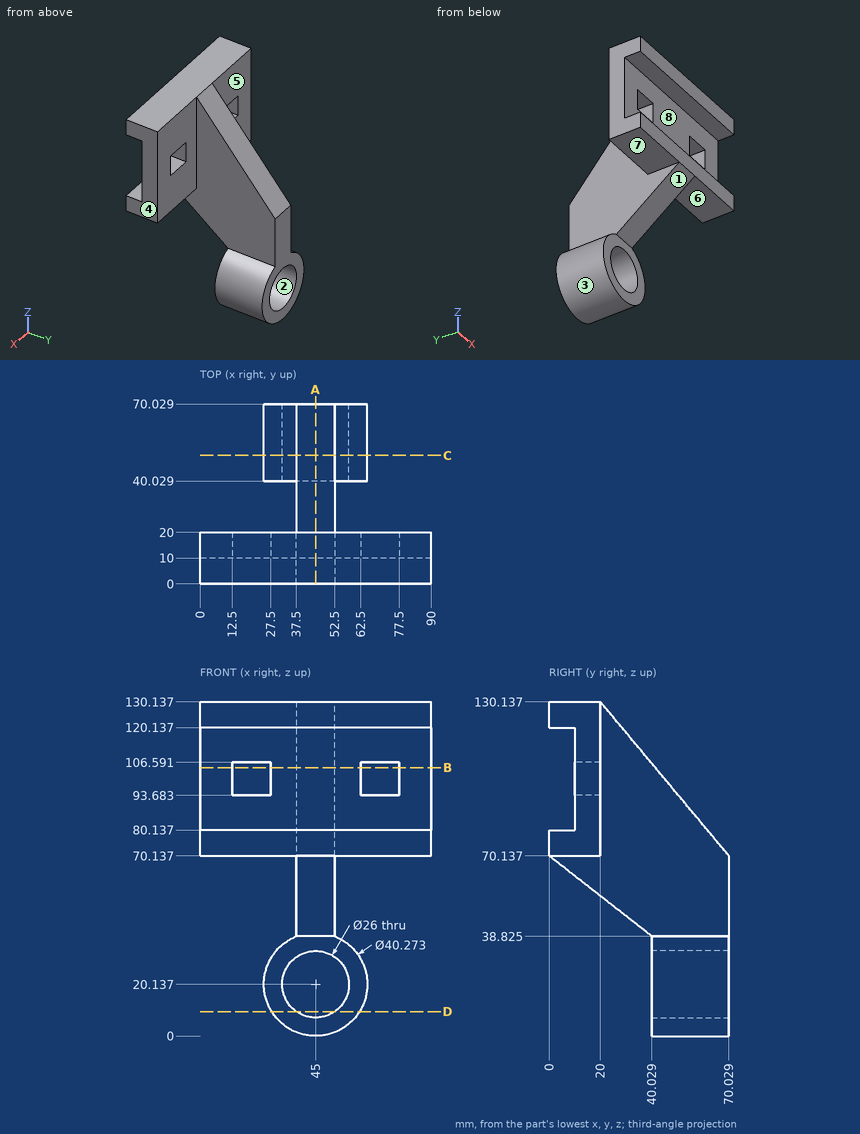
For this review, use the dimensioned drawing (mm, ordinates from the lowest corner) and the shaded views. A direction names the side the tool comes from. Round coordinates to 2 decimals unless told otherwise and drop trailing zeros. Write each loop counter-clockwise with the first axis right and the second up, starting at its lowest first coordinate (ties: lowest second). Pieces come first, ordered by that corner, then holes. Notation, with made-up numbers: (82.25, -25.75) -> (140.25, -25.75) arc R20 ccw to (140.25, -21.75) -> close; hole circle Ø6 at (3, 9.5). An arc over 180 degrees is marked (long way). Use one line per item in the form item = value.
Q1. Consider section D-D (z = 9.5). State the section outline as (x, y) points.
Resolved:
outline = (27.9, 40.03) -> (37.53, 40.03) -> (37.53, 70.03) -> (27.9, 70.03) -> close; (52.47, 40.03) -> (62.1, 40.03) -> (62.1, 70.03) -> (52.47, 70.03) -> close
Q2. Consider section C-C (y = 50). State the section outline as (x, z) points (1 decimal), then the cut area to 3 significant figures.
Resolved:
outline = (37.5, 38.8) arc R20.1 ccw (long way) to (52.5, 38.8) -> (52.5, 94.2) -> (37.5, 94.2) -> close; hole circle Ø26 at (45, 20.1)
area = 1,560 mm²
Q3. Machinability: for the marked faces 5, 6, 7 and 8, which of the approach directions +Z, -Z, +X, -X, +Y, -Y give a long, thin tool a straight path to every point of the face, cutting with its end or side? Answer none if there is none.
Resolved:
face_5 = +Z, -Z, -X, +Y
face_6 = -Z, +X, +Y, -Y
face_7 = -Z, -X, +Y, -Y
face_8 = +X, -X, -Y
Q4. To check wall thickness, follow probe 1 along X at (y, z) = (46.5, 20); probe 2 along Z at (x, y) = (22.5, 17); probe 3 along Y at (x, z) = (35.5, 109). State the ranges of each line that lie inside material, in increasing order. Write a range as from..to.
Resolved:
probe_1 = 24.86..32, 58..65.14
probe_2 = 70.14..93.68, 106.59..130.14
probe_3 = 10..20
Q5. Consider section B-B (z = 104.5). State the section outline as (x, y) points.
Resolved:
outline = (0, 10) -> (12.5, 10) -> (12.5, 20) -> (0, 20) -> close; (27.5, 10) -> (62.5, 10) -> (62.5, 20) -> (52.5, 20) -> (52.5, 41.38) -> (37.5, 41.38) -> (37.5, 20) -> (27.5, 20) -> close; (77.5, 10) -> (90, 10) -> (90, 20) -> (77.5, 20) -> close
Q6. Clearance check with flat-ended pins moving along their axes: pin 1 Ø2 at (x, y) = (56.5, 16) entering from -Z; pin 2 Ø6 at (x, z) = (26, 115) entering from -Y; pin 3 Ø8 at (x, y) = (35, 7) entering from -Z; pin 4 Ø15.5 at (x, z) = (45, 20.14) entering from +Y. State where each tip first meets the part, or that it passes through.
Resolved:
pin_1 = 70.14
pin_2 = 10
pin_3 = 62.22
pin_4 = through
Q7. Consider section A-A (x = 45). State the section outline as (y, z) points (1 decimal), then the cut area to 3 significant figures.
Resolved:
outline = (0, 70.1) -> (40, 38.8) -> (40, 33.1) -> (70, 33.1) -> (70, 70.1) -> (20, 130.1) -> (0, 130.1) -> (0, 120.1) -> (10, 120.1) -> (10, 80.1) -> (0, 80.1) -> close; (40, 0) -> (70, 0) -> (70, 7.1) -> (40, 7.1) -> close
area = 4,250 mm²
Q8. The part is to be moulded in two halves that separate along X. For the marked faces 1, 2, 3 and 4, say which applies: released by +X, released by -X, zero draft, split by the parting line, or undercut.
Resolved:
face_1 = zero draft
face_2 = undercut
face_3 = split by the parting line
face_4 = released by +X
